Could you check a few things on this model? Use its own coordinates, in mm. Coordinates: 2 decimals unless noted, no trailing zeros. Write each loop counter-clockwise with the first axis right and the second up, starting at its lowest first coordinate (ties: lowest second). Pieces come first, ordered by that corner, then holes. Notation, with made-up numbers: (73, 9.25) - (131, 9.25) arc R35 ccw to (131, 43.25) - close; hole circle Ø4 at (73, 32). An arc over 180 degrees is marked (long way). Answer as a JSON object with one key per item and string values. Group by question number.
1) Please list where these lines run through material, in increasing order: line 1 along Y through (x, z) = (10, -0.4); line 2 along X through (y, z) = (-30, -1.3); line 3 along Y through (x, z) = (30, -0.8).
2) If we section it at D-D (x = 10): Write out the boundary of the cut face in (y, z).
3) Will these pins go through, and if not, where does the flat tip stop? pin 1 Ø3.5 at (x, y) = (10, -30) entering from +Z; pin 2 Ø4 at (x, y) = (35.5, -22.5) entering from +Z.
4) If we section it at C-C (z = -1.15): Write out the boundary of the cut face in (x, y), plus the area to 3 significant figures.
5) If we section it at A-A (x = 30): Write out the boundary of the cut face in (y, z).
6) We'd pull the mould along Y, two halves only. Please class faces 1 (the flat face through (30, -10, -1)), 2 (the cylindrical face through (32.027, -31.859, -0.986)), 3 (the cylindrical face through (8.52, -12.32, -0.99)), 4 (the flat face through (1, -39, -1)): released by +Y, released by -Y, zero draft, split by the parting line, or undercut.
7) If we section it at B-B (y = -10): Write out the boundary of the cut face in (x, z), plus the area to 3 significant figures.
```python
from build123d import *

# Parameters (mm, degrees)
EXTRUDE_1_DEPTH   = 2
HOLE_WIZARD_M51_D = 5.5
CHAMFER_1_SIZE    = 2


with BuildPart() as part:
    # Эскиз1 → Бобышка-Вытянуть1 (new body)
    with BuildSketch(Plane(origin=(0, 0, 0), x_dir=(1, 0, 0), z_dir=(0, 0, -1))):
        Polygon((0, 0), (0, 40), (40, 40), (40, 20), (20, 0), align=None)
    extrude(amount=EXTRUDE_1_DEPTH)

    # Отверстие с зазором M51 (through all)
    with Locations(Plane(origin=(0, 0, -2), x_dir=(1, 0, 0), z_dir=(0, 0, -1))):
        with Locations((10, 30), (10, 10), (30, 30)):
            Hole(HOLE_WIZARD_M51_D / 2)

    # Фаска1
    chamfer_1_edges = [part.edges().sort_by_distance(p)[0] for p in [
        (0, 0, -1),
        (0, -40, -1),
        (40, -40, -1),
    ]]
    chamfer(chamfer_1_edges, length=CHAMFER_1_SIZE)


solid = part.part
```
Here are the results:
{
 "1": {"line 1": "y = -40 to -32.75, -27.25 to -12.75, -7.25 to 0", "line 2": "x = 0 to 7.25, 12.75 to 27.25, 32.75 to 40", "line 3": "y = -40 to -32.75, -27.25 to -10"},
 "2": {"outline": "(-40, -2) - (-32.75, -2) - (-32.75, 0) - (-40, 0) - close; (-27.25, -2) - (-12.75, -2) - (-12.75, 0) - (-27.25, 0) - close; (-7.25, -2) - (0, -2) - (0, 0) - (-7.25, 0) - close"},
 "3": {"pin 1": "passes through", "pin 2": "stops at z = 0"},
 "4": {"outline": "(0, -38) - (2, -40) - (38, -40) - (40, -38) - (40, -20) - (20, 0) - (2, 0) - (0, -2) - close; hole circle Ø5.5 at (10, -30); hole circle Ø5.5 at (10, -10); hole circle Ø5.5 at (30, -30)", "area": "1,320 mm²"},
 "5": {"outline": "(-40, -2) - (-32.75, -2) - (-32.75, 0) - (-40, 0) - close; (-27.25, -2) - (-10, -2) - (-10, 0) - (-27.25, 0) - close"},
 "6": {"face 1": "released by +Y", "face 2": "undercut", "face 3": "undercut", "face 4": "released by -Y"},
 "7": {"outline": "(0, -2) - (7.25, -2) - (7.25, 0) - (0, 0) - close; (12.75, -2) - (30, -2) - (30, 0) - (12.75, 0) - close", "area": "49.0 mm²"}
}
